Autodesk Inventor part; units mm, degrees
ref_plane "YZ Plane" through (0, 0, 0) normal (1, 0, 0) x (0, 1, 0)
ref_plane "XZ Plane" through (0, 0, 0) normal (0, 1, 0) x (-1, 0, 0)
ref_plane "XY Plane" through (0, 0, 0) normal (0, 0, 1) x (1, 0, 0)
sketch "Sketch1" plane through (0, 0, 0) normal (0, 0, 1) x (1, 0, 0)
  line L0 (0, 0) -> (12.7, 0)
  line L1 (12.7, 0) -> (12.7, 35.56)
  line L2 (12.7, 35.56) -> (0, 35.56)
  line L3 (0, 35.56) -> (0, 0)
  line L4 (1.27, 34.29) -> (11.43, 34.29)
  line L5 (11.43, 34.29) -> (11.43, 1.27)
  line L6 (11.43, 1.27) -> (1.27, 1.27)
  line L7 (1.27, 1.27) -> (1.27, 34.29)
  dimension "d0" = 35.56
  dimension "d1" = 12.7
  dimension "d2" = 1.27
extrude "Extrusion1" add sketch "Sketch1" along normal blind 203.2
sketch "Sketch2" plane through (12.7, 0, 0) normal (1, 0, 0) x (0, 0, -1)
  line L0 (-168.1044, 17.78) -> (-15.152, 17.78) construction
  line L1 (0, 0) -> (-203.2, 0) construction
  line L2 (-203.2, 0) -> (-203.2, 35.56)
  line L3 (0, 0) -> (0, 35.56)
  point P0 (-177.8, 17.78)
  point P1 (-25.4, 17.78)
  dimension "d5" = 17.78
  dimension "d6" = 25.4
  dimension "d7" = 25.4
hole "Hole1" at (12.7, 17.78, 177.8) at (12.7, 17.78, 25.4) direction (-1, 0, 0) diameter 3.2639 end through all
sketch "Sketch3" plane through (12.7, 0, 0) normal (1, 0, 0) x (0, 0, -1)
  circle A0 centre (-177.8, 17.78) radius 1.632
  circle A1 centre (-25.4, 17.78) radius 1.632
  line L0 (-214.4228, 17.78) -> (16.7128, 17.78) construction
  point P0 (0, 0)
  point P1 (-177.8, 17.78)
  point P2 (-25.4, 17.78)
  point P3 (-139.7, 17.78)
  point P4 (-63.5, 17.78)
  dimension "d18" = 38.1
  dimension "d19" = 38.1
hole "Hole2" at (12.7, 17.78, 139.7) at (12.7, 17.78, 63.5) direction (-1, 0, 0) diameter 6.5278 end through all
sketch "Sketch4" plane through (0, 35.56, 0) normal (0, 1, 0) x (1, 0, 0)
  line L0 (6.35, 23.2485) -> (6.35, -226.9955) construction
  line L1 (12.7, 0) -> (12.7, -203.2) construction
  line L2 (12.7, 0) -> (0, 0)
  line L3 (0, 0) -> (0, -203.2)
  line L4 (12.7, -203.2) -> (0, -203.2)
  line L5 (12.7, 0) -> (12.7, -203.2)
  point P0 (0, 0)
  point P1 (6.35, -31.75)
  point P2 (6.35, -171.45)
  dimension "d27" = 6.35
  dimension "d28" = 31.75
  dimension "d29" = 31.75
hole "Hole3" at (6.35, 35.56, 31.75) at (6.35, 35.56, 171.45) direction (0, -1, 0) diameter 3.2512 end through all
sketch "Sketch5" plane through (0, 35.56, 0) normal (0, 1, 0) x (1, 0, 0)
  line L0 (-85.4565, -101.6) -> (166.25, -101.6) construction
  line L1 (12.7, 0) -> (0, 0) construction
  line L2 (6.35, 16.7541) -> (6.35, -272.8802) construction
  line L3 (0, 0) -> (0, -203.2) construction
  line L4 (-54.5343, -133.35) -> (67.2343, -133.35) construction
  line L5 (-32.5067, -69.85) -> (120.6854, -69.85) construction
  line L6 (12.7, -203.2) -> (0, -203.2) construction
  point P0 (6.35, -69.85)
  point P1 (6.35, -133.35)
  dimension "d37" = 101.6
  dimension "d38" = 6.35
  dimension "d39" = 31.75
  dimension "d40" = 31.75
hole "Hole4" at (6.35, 35.56, 69.85) at (6.35, 35.56, 133.35) direction (0, -1, 0) diameter 3.175 end through all
properties part number "000101-1"
For this review, take the finished solid that the model builds, in its own axes (mm). A direction names the side the tool comes from. Give positions to 0.01 mm unless a question says otherwise; leave off trailing zeros. Loops run counter-clockwise (first coordinate to the right, second up) from the corner with the lowest first, then second, coordinate; pieces in that order, holes last.
Item 1: Take a section at A-A, the plane y = 29. State the section outline as (x, z) points, and give its area (3 significant figures).
Item 2: Take a section at B-B, the plane z = 139.7. State the section outline as (x, y) points.
Item 3: Insertion check: pin 1 (5 mm diameter, centred on x = 8.5, z = 131, fed in from -Y). The pin has a flat end and moves straight along its axis. Give the tip position at first contact, or say it passes through.
Item 4: Tool access review of faces 1 (the cylindrical face through (6.279, 0.626, 169.826)), 2 (the flat face through (11.43, 18, 100)): name each direction out of +Z, -Z, +X, -X, +Y, -Y from which nothing blocks a thin tool from reaching the whole face with its end or side.
Item 5: For line 1 along Z through (x, y) = (6.35, 35.3); line 2 along X through (y, z) = (18, 55); line 3 along Y through (x, z) = (6.5, 76), list the stretches that pass through material, from the lowest coordinate up.
Item 6: Draft analysis for pull direction Z (two halves, no side actions). For faces 3 (the flat face through (1.27, 18, 100)), 4 (the flat face through (1, 19, 203.2)), 5 (the cylindrical face through (5.873, 0.626, 134.864)), state which applies: +Z half, -Z half, draft (parallel to the pull), parting line (faces both ways), or undercut.
Item 7: Take a section at C-C, the plane z = 20.5. State the section outline as (x, y) points, and give its area (3 significant figures).
Calculated:
1. outline: (0, 0) - (1.27, 0) - (1.27, 203.2) - (0, 203.2) - close; (11.43, 0) - (12.7, 0) - (12.7, 203.2) - (11.43, 203.2) - close
1. area: 516 mm2
2. outline: (0, 0) - (12.7, 0) - (12.7, 14.52) - (11.43, 14.52) - (11.43, 1.27) - (1.27, 1.27) - (1.27, 14.52) - (0, 14.52) - close; (0, 21.04) - (1.27, 21.04) - (1.27, 34.29) - (11.43, 34.29) - (11.43, 21.04) - (12.7, 21.04) - (12.7, 35.56) - (0, 35.56) - close
3. pin 1: stops at y = 0
4. face 1: +Y, -Y
4. face 2: +Z, -Z
5. line 1: z = 0 to 30.12, 33.38 to 68.26, 71.44 to 131.76, 134.94 to 169.82, 173.08 to 203.2
5. line 2: x = 0 to 1.27, 11.43 to 12.7
5. line 3: y = 0 to 1.27, 34.29 to 35.56
6. face 3: draft
6. face 4: +Z half
6. face 5: undercut
7. outline: (0, 0) - (12.7, 0) - (12.7, 35.56) - (0, 35.56) - close; hole (1.27, 1.27) - (11.43, 1.27) - (11.43, 34.29) - (1.27, 34.29) - close
7. area: 116 mm2
